Source: CAD feature listing. Evaluate the final solid. Frame: model axes, mm. A direction names the side the tool comes from. Give positions to 0.01 mm unless a question says otherwise; leave off trailing zeros.
from build123d import *

# Parameters (mm, degrees)
SKETCH1_R               = 127
SKETCH1_R_2             = 12.5
BOSS_EXTRUDE1_DEPTH     = 1046
SKETCH3_R               = 12.5
BOSS_EXTRUDE2_DEPTH     = 584
BOSS_EXTRUDE4_START     = 6
SKETCH4_R               = 75
SKETCH4_R_2             = 12.5
BOSS_EXTRUDE4_DEPTH     = 6
SKETCH6_R               = 75
BOSS_EXTRUDE5_DEPTH     = 6
CUT_EXTRUDE1_DEPTH      = 1138.271735339
CUT_EXTRUDE1_DEPTH_BACK = 1138.271735339
SKETCH7_R               = 6
CUT_EXTRUDE2_DEPTH      = 1132.347426744
CUT_EXTRUDE2_DEPTH_BACK = 1132.347426744
SKETCH8_R               = 10


with BuildPart() as part:
    # Sketch1 → Boss-Extrude1 (new body)
    with BuildSketch(Plane.XY):
        Circle(SKETCH1_R)
        Circle(SKETCH1_R_2, mode=Mode.SUBTRACT)
    extrude(amount=BOSS_EXTRUDE1_DEPTH)

    # Sketch3 → Boss-Extrude2 (add, symmetric)
    with BuildSketch(Plane.XY.offset(533)):
        Circle(SKETCH3_R)
    extrude(amount=BOSS_EXTRUDE2_DEPTH, both=True)

    # Sketch4 → Boss-Extrude4 (add)
    with BuildSketch(Plane.XY.offset(1046).offset(BOSS_EXTRUDE4_START)):
        Circle(SKETCH4_R)
        Circle(SKETCH4_R_2, mode=Mode.SUBTRACT)
    extrude(amount=-BOSS_EXTRUDE4_DEPTH)

    # Sketch6 → Boss-Extrude5 (add)
    with BuildSketch(Plane(origin=(0, 0, 0), x_dir=(-1, 0, 0), z_dir=(0, 0, -1))):
        with Locations(Location((0, 0, 0), (0, 0, 180))):
            Circle(SKETCH6_R)
    extrude(amount=BOSS_EXTRUDE5_DEPTH)

    # Sketch7 → Cut-Extrude1 (cut, two sides: drawn at the far end of the back side and taken through both)
    with BuildSketch(Plane(origin=(0, 0, -6), x_dir=(-1, 0, 0), z_dir=(0, 0, -1)).offset(-CUT_EXTRUDE1_DEPTH_BACK)):
        with Locations((0, 55)):
            Circle(SKETCH7_R)
        with Locations((38.890872965, 38.890872965)):
            Circle(SKETCH7_R)
        with Locations((55, 0)):
            Circle(SKETCH7_R)
        with Locations((38.890872965, -38.890872965)):
            Circle(SKETCH7_R)
        with Locations((0, -55)):
            Circle(SKETCH7_R)
        with Locations((-38.890872965, -38.890872965)):
            Circle(SKETCH7_R)
        with Locations((-55, 0)):
            Circle(SKETCH7_R)
        with Locations((-38.890872965, 38.890872965)):
            Circle(SKETCH7_R)
    extrude(amount=CUT_EXTRUDE1_DEPTH + CUT_EXTRUDE1_DEPTH_BACK, mode=Mode.SUBTRACT)

    # Sketch8 → Cut-Extrude2 (cut, two sides: drawn at the far end of the back side and taken through both)
    with BuildSketch(Plane(origin=(0, 0, 0), x_dir=(-1, 0, 0), z_dir=(0, 0, -1)).offset(-CUT_EXTRUDE2_DEPTH_BACK)):
        with Locations((0, 127)):
            Circle(SKETCH8_R)
        with Locations((39.245158286, 120.784177569)):
            Circle(SKETCH8_R)
        with Locations((74.648727041, 102.745158286)):
            Circle(SKETCH8_R)
        with Locations((102.745158286, 74.648727041)):
            Circle(SKETCH8_R)
        with Locations((120.784177569, 39.245158286)):
            Circle(SKETCH8_R)
        with Locations((127, 0)):
            Circle(SKETCH8_R)
        with Locations((120.784177569, -39.245158286)):
            Circle(SKETCH8_R)
        with Locations((102.745158286, -74.648727041)):
            Circle(SKETCH8_R)
        with Locations((74.648727041, -102.745158286)):
            Circle(SKETCH8_R)
        with Locations((39.245158286, -120.784177569)):
            Circle(SKETCH8_R)
        with Locations((0, -127)):
            Circle(SKETCH8_R)
        with Locations((-39.245158286, -120.784177569)):
            Circle(SKETCH8_R)
        with Locations((-74.648727041, -102.745158286)):
            Circle(SKETCH8_R)
        with Locations((-102.745158286, -74.648727041)):
            Circle(SKETCH8_R)
        with Locations((-120.784177569, -39.245158286)):
            Circle(SKETCH8_R)
        with Locations((-127, 0)):
            Circle(SKETCH8_R)
        with Locations((-120.784177569, 39.245158286)):
            Circle(SKETCH8_R)
        with Locations((-102.745158286, 74.648727041)):
            Circle(SKETCH8_R)
        with Locations((-74.648727041, 102.745158286)):
            Circle(SKETCH8_R)
        with Locations((-39.245158286, 120.784177569)):
            Circle(SKETCH8_R)
    extrude(amount=CUT_EXTRUDE2_DEPTH + CUT_EXTRUDE2_DEPTH_BACK, mode=Mode.SUBTRACT)


solid = part.part
1) Section query A-A on z = 856. State how many separate pieces and enclosed holes the cut face has, and give its area (3 significant figures).
Checks:
separate pieces: 1
enclosed holes: 8
area: 46,700 mm2
2) Ray query, L1, parallel to X at y = -1.5, z = 1038; L2, parallel to Y at x = 0, z = 381; L3, parallel to Y at x = 96, z = 705. Return the intervals inside material, ascending.
Checks:
L1: x = -117.11 to -60.81, -49.19 to 49.19, 60.81 to 117.11
L2: y = -117 to -61, -49 to 49, 61 to 117
L3: y = -83.14 to -82.03, -67.27 to 67.27, 82.03 to 83.14
3) Reachability of faces 1 (the face through (-35.952, 111.342, 530.322)), 2 (the face through (11.923, 3.755, 1084.955)), 3 (the face through (11.923, 3.755, -28.185)) from +Z, -Z, +X, -X, +Y, -Y: full face, straight path, thin tool, end or side. Return the list, or none.
Checks:
face 1: +Z, -Z
face 2: +Z
face 3: -Z
4) First-contact query: pin 1 Ø1 at (y, z) = (-4.5, 543.5) entering from +X; pin 2 Ø15.5 at (x, y) = (38.89, -38.89) entering from -Z; pin 3 Ø1 at (x, z) = (6.5, 387.5) entering from +Y; pin 4 Ø11 at (x, y) = (0, 55) entering from -Z. Flat tips, straight axial feed; report the tip coordinate or a pass-through.
Checks:
pin 1: stops at x = 118.34
pin 2: stops at z = -6
pin 3: stops at y = 119.86
pin 4: passes through
5) Pull-direction query (Y, two-part tool) for faces 4 (the face through (117, 0, 530)), 5 (the face through (-117, 0, 530)), 6 (the face through (125.415, -20.005, 515.678)), 7 (the face through (-19.73, 125.46, 515.68)); classes: +Y half, -Y half, draft (parallel to the pull), parting line (faces both ways), or undercut.
Checks:
face 4: undercut
face 5: undercut
face 6: -Y half
face 7: +Y half
